Geometry: final body of the model. Coordinates: model frame, mm. A direction names the side the tool comes from. Give positions to 0.01 mm unless a question says otherwise; leave off trailing zeros. Order: outer loops, then holes, each group sorted by start corner. A loop starts at its lowest first (then second) coordinate and runs counter-clockwise, first axis right, second up. Notation, with made-up numbers: (61, 57) -> (69, 57) arc R32 ccw to (69, 96) -> close; hole circle Ø10 at (-37.75, 13). An arc over 180 degrees is marked (long way). Answer in a Markdown table with one row per item. Add a question column.
Q1. Cut plane B-B on x = -40. Return the cut outline in (y, z), and give its area (3 significant figures).
Q2. Cut plane A-A on z = 14.5. Return the cut outline in (x, y).
Q3. Contact query for flat-ended pins moving along their axis: P1, Ø24.5, axis at x = -45, y = -31.5, coming from the -Z side; P2, Ø23.5, axis at y = -31, z = 73, coming from the +X side; P3, Ø5.5, axis at y = -35, z = 67.5, coming from the -X side. Output: stop coordinate, or through.
Q4. Pull-direction query (Y, two-part tool) for faces 6 (the face through (-30, -49, 50.468)), 7 (the face through (8.872, -7.929, 27.419)), 8 (the face through (1.641, -13.807, 66.211)); classes: +Y half, -Y half, draft (parallel to the pull), parting line (faces both ways), or undercut.
Q5. Cut plane C-C on y = -33. Return the cut outline in (x, z), and give its area (3 significant figures).
Q6. Set-up query: faces 1 (the face through (-67.823, -19, 69)), 2 (the face through (-65.283, -20, 66)), 3 (the face through (3.418, -11.992, 68.751)), 4 (the face through (7.657, -33, 69)), 5 (the face through (-63.801, -39.194, 69.27)). Return all of +Z, -Z, +X, -X, +Y, -Y with unobstructed straight access to the full face (end or side cutting, diameter ignored); none if empty.
Q7. Line query: line 1 along Y through (x, z) = (-31.5, 36.5); line 2 along Z through (x, y) = (8, -29); line 3 along X through (y, z) = (-25.5, 38.5). Output: solid intervals per line, ascending. Write a range as from..to.
Q8. Cut plane D-D on z = 53. Return the cut outline in (x, y).
from build123d import *

# Parameters (mm, degrees)
F0_W     = 91.7905736715
F0_H     = 46.7539317906
F1_DEPTH = 52.07
F2_R     = 26.3680405282
F3_W     = 75.4797728732
F3_H     = 35.4631096125
F4_DEPTH = 25.4
F5_DEPTH = 11.684
F6_R     = 14.1038356314
F7_R     = 14.097
F8_T     = -2.54


with BuildPart() as f1:
    # F0 (on Front) → F1 (new body)
    with BuildSketch(Plane.XZ):
        with Locations((-29.504111968, 27.0913075656)):
            Rectangle(F0_W, F0_H)
    extrude(amount=F1_DEPTH)

    # F2
    f2_edges = [f1.edges().sort_by_distance(p)[0] for p in [
        (-75.399399, -52.07, 27.091308),
        (16.391175, 0, 27.091308),
    ]]
    fillet(f2_edges, radius=F2_R)

    # F3 (on face) → F4 (join)
    with BuildSketch(Plane.XY.offset(50.4682734609)):
        with Locations((-30.0831585191, -25.7032476366)):
            Rectangle(F3_W, F3_H)
    extrude(amount=F4_DEPTH)

    # F5 (add): a face of the model
    f5_faces = [f1.faces().sort_by_distance(p)[0] for p in [
        (-30.0831585191, -25.7032476366, 75.8682734609),
    ]]
    extrude(f5_faces, amount=F5_DEPTH)

    # F6
    f6_edges = [f1.edges().sort_by_distance(p)[0] for p in [
        (-67.823045, -43.434802, 69.010273),
    ]]
    fillet(f6_edges, radius=F6_R)

    # F7
    f7_edges = [f1.edges().sort_by_distance(p)[0] for p in [
        (7.656728, -7.971693, 69.010273),
    ]]
    fillet(f7_edges, radius=F7_R)

    # F8
    f8_openings = [f1.faces().sort_by_distance(p)[0] for p in [
        (-29.504112, -26.035, 3.714342),
    ]]
    offset(amount=F8_T, openings=f8_openings, kind=Kind.INTERSECTION)


solid = f1.part
Completed:
| question | item | result |
|---|---|---|
| 1 | outline | (-52.07, 3.71) -> (-49.53, 3.71) -> (-49.53, 47.93) -> (-40.89, 47.93) -> (-40.89, 85.01) -> (-10.51, 85.01) -> (-10.51, 47.93) -> (-2.54, 47.93) -> (-2.54, 3.71) -> (0, 3.71) -> (0, 50.47) -> (-7.97, 50.47) -> (-7.97, 87.55) -> (-43.43, 87.55) -> (-43.43, 50.47) -> (-52.07, 50.47) -> close |
| 1 | area | 545 mm² |
| 2 | outline | (-75.4, -25.7) arc R26.37 ccw to (-49.03, -52.07) -> (16.39, -52.07) -> (16.39, -26.37) arc R26.37 ccw to (-9.98, 0) -> (-75.4, 0) -> close; hole (-72.86, -25.7) arc R23.83 ccw to (-49.03, -49.53) -> (13.85, -49.53) -> (13.85, -26.37) arc R23.83 ccw to (-9.98, -2.54) -> (-72.86, -2.54) -> close |
| 3 | P1 | stops at z = 47.93 |
| 3 | P2 | stops at x = 7.66 |
| 3 | P3 | stops at x = -67.52 |
| 4 | face 6 | draft |
| 4 | face 7 | +Y half |
| 4 | face 8 | undercut |
| 5 | outline | (-74.37, 3.71) -> (-71.71, 3.71) -> (-71.71, 47.93) -> (-64.69, 47.93) -> (-64.69, 85.01) -> (5.12, 85.01) -> (5.12, 47.93) -> (13.85, 47.93) -> (13.85, 3.71) -> (16.39, 3.71) -> (16.39, 50.47) -> (7.66, 50.47) -> (7.66, 87.55) -> (-67.34, 87.55) -> (-67.34, 50.47) -> (-74.37, 50.47) -> close |
| 5 | area | 653 mm² |
| 6 | face 1 | +Z, -X, +Y, -Y |
| 6 | face 2 | -Z |
| 6 | face 3 | +Z, +X, +Y |
| 6 | face 4 | +Z, +X, +Y, -Y |
| 6 | face 5 | +Z, -X, -Y |
| 7 | line 1 | y = -52.07..-49.53, -2.54..0 |
| 7 | line 2 | z = 47.93..50.47 |
| 7 | line 3 | x = -75.4..-72.86, 13.84..16.38 |
| 8 | outline | (-67.82, -29.33) arc R14.1 ccw to (-53.72, -43.43) -> (7.66, -43.43) -> (7.66, -22.07) arc R14.1 ccw to (-6.44, -7.97) -> (-67.82, -7.97) -> close; hole (-65.28, -29.33) arc R11.56 ccw to (-53.72, -40.89) -> (5.12, -40.89) -> (5.12, -22.07) arc R11.56 ccw to (-6.44, -10.51) -> (-65.28, -10.51) -> close |
